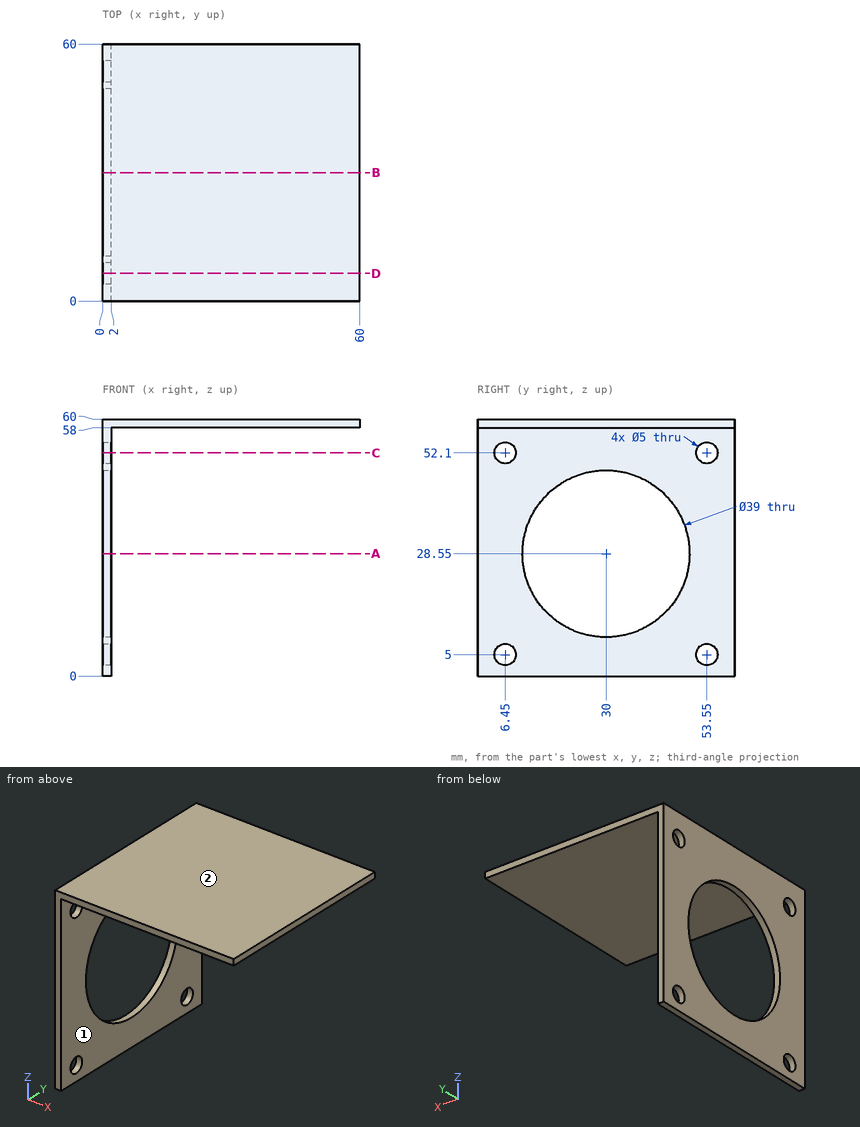
Input: dimensioned drawing with shaded views. Units: mm. Origin: part minimum x, y, z. A direction names the side the tool comes from. Give positions to 0.01 mm unless a question says otherwise; leave off trailing zeros. Write each loop counter-clockwise with the first axis right and the second up, starting at its lowest first coordinate (ties: lowest second). Pieces come first, ordered by that corner, then holes. Notation, with made-up numbers: (-26.75, 52.25) - (24.25, 52.25) arc R24 ccw to (24.25, 68.25) - close; hole circle Ø9 at (22, 34). An arc over 180 degrees is marked (long way). Write item = value, one per line. Start each with the question number.
1) Cut plane C-C (z = 52.1). Return loops of the section in (x, y).
2) Reachability of the marked faces 1 and 2 from +Z, -Z, +X, -X, +Y, -Y: full face, straight path, thin tool, end or side. Return the list, or none.
3) Cut plane D-D (y = 6.45). Return loops of the section in (x, z), and give its area (3 significant figures).
4) Cut plane B-B (y = 30). Return loops of the section in (x, z).
5) Cut plane A-A (z = 28.55). Return loops of the section in (x, y), and give its area (3 significant figures).
6) Pin query (flat end, axial travel): pin 1 (4 mm diameter, centred on y = 6.45, z = 5, fed in from +X); pin 2 (8 mm diameter, centred on y = 53.55, z = 52.1, fed in from -X); pin 3 (3 mm diameter, centred on x = 7, y = 34, fed in from -Z); pin 4 (6 mm diameter, centred on y = 6.45, z = 52.1, fed in from +X). Return the tip coordinate at first contact, or that it passes through.
7) Material intervals for L1, parallel to Y at x = 1.1, z = 5; L2, parallel to X at y = 21, z = 51; L3, parallel to Z at x = 29.5, y = 40, sorted ascending. Write a range as [from, to].
Answers follow:
q1.outline = (0, 0) - (2, 0) - (2, 3.95) - (0, 3.95) - close; (0, 8.95) - (2, 8.95) - (2, 51.05) - (0, 51.05) - close; (0, 56.05) - (2, 56.05) - (2, 60) - (0, 60) - close
q2.face_1 = -Z, +X, +Y, -Y
q2.face_2 = +Z, +X, -X, +Y, -Y
q3.outline = (0, 0) - (2, 0) - (2, 2.5) - (0, 2.5) - close; (0, 7.5) - (2, 7.5) - (2, 49.6) - (0, 49.6) - close; (0, 54.6) - (2, 54.6) - (2, 58) - (60, 58) - (60, 60) - (0, 60) - close
q3.area = 216 mm^2
q4.outline = (0, 0) - (2, 0) - (2, 9.05) - (0, 9.05) - close; (0, 48.05) - (2, 48.05) - (2, 58) - (60, 58) - (60, 60) - (0, 60) - close
q5.outline = (0, 0) - (2, 0) - (2, 10.5) - (0, 10.5) - close; (0, 49.5) - (2, 49.5) - (2, 60) - (0, 60) - close
q5.area = 42.0 mm^2
q6.pin_1 = through
q6.pin_2 = 0
q6.pin_3 = 58
q6.pin_4 = 2
q7.L1 = [0, 3.95], [8.95, 51.05], [56.05, 60]
q7.L2 = [0, 2]
q7.L3 = [58, 60]
